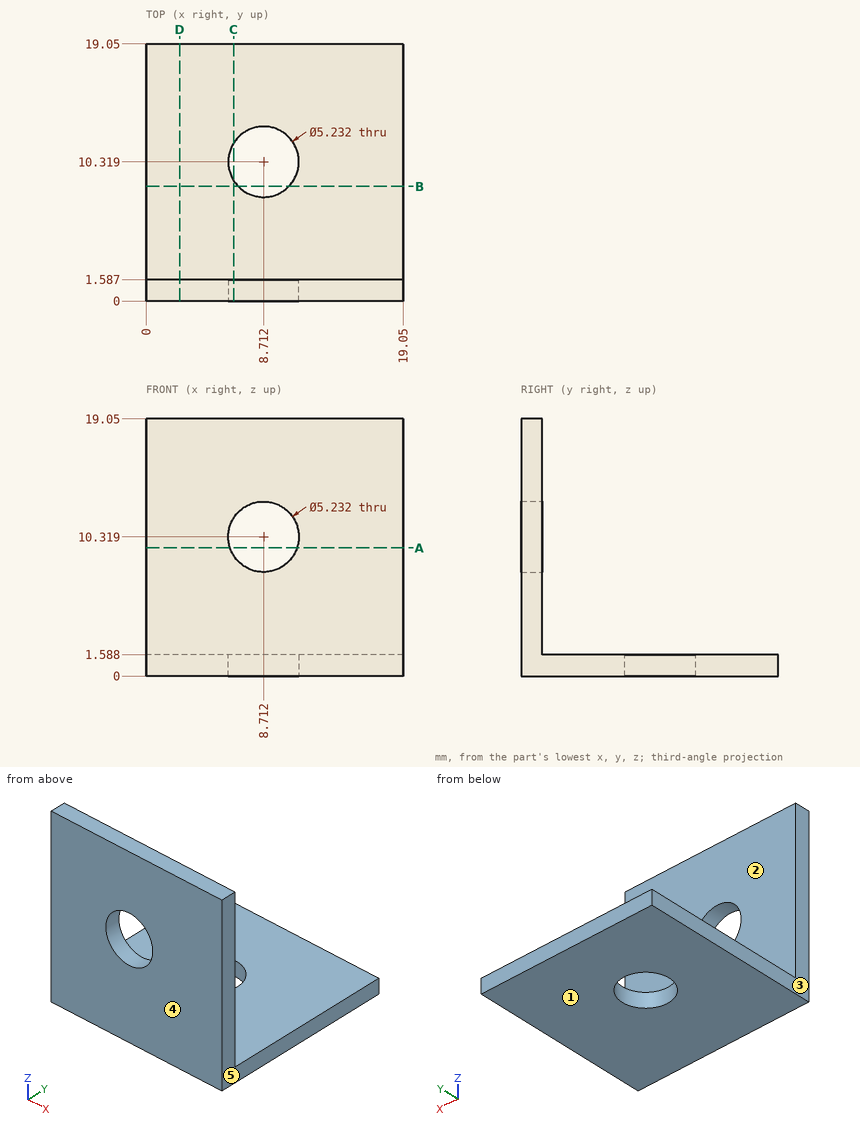
Part print with two shaded views. Sizes in mm from the minimum x, y, z corner. A direction names the side the tool comes from. Round coordinates to 2 decimals unless told otherwise and drop trailing zeros. Order: outer loops, then holes, each group sorted by start corner. A loop starts at its lowest first (then second) coordinate and runs counter-clockwise, first axis right, second up. Notation, with made-up numbers: (43.25, 35.5) -> (89.25, 35.5) arc R23 ccw to (89.25, 57.5) -> close; hole circle Ø7 at (13.25, 21.5). An arc over 180 degrees is marked (long way). One line per question, with ' | ' between items.
Q1. Slice it at A-A (z = 9.5). Write the cut outline in (x, y).
Completed:
outline: (0, 0) -> (6.23, 0) -> (6.23, 1.59) -> (0, 1.59) -> close; (11.2, 0) -> (19.05, 0) -> (19.05, 1.59) -> (11.2, 1.59) -> close
Q2. Slice it at C-C (x = 6.5). Give the number of separate pieces and of enclosed holes in the cut face.
Completed:
separate pieces: 3 | enclosed holes: 0
Q3. Slice it at D-D (x = 2.5). Write the cut outline in (y, z).
Completed:
outline: (0, 0) -> (19.05, 0) -> (19.05, 1.59) -> (1.59, 1.59) -> (1.59, 19.05) -> (0, 19.05) -> close
Q4. Drop flat-ended pins along their axis: pin 1 (8.5 mm diameter, centred on x = 13, y = 11, fed in from +Z); pin 2 (6 mm diameter, centred on x = 15, z = 12.5, fed in from +Y). Give the stop position or say it passes through.
Completed:
pin 1: stops at z = 1.59 | pin 2: stops at y = 1.59
Q5. Two-plate mould, pull along X, no slides. Class the marked faces 3, 4 and 5: released by +X, released by -X, zero draft, split by the parting line, or undercut.
Completed:
face 3: released by -X | face 4: zero draft | face 5: released by +X
Q6. Slice it at B-B (y = 8.5). Write the cut outline in (x, z).
Completed:
outline: (0, 0) -> (6.83, 0) -> (6.83, 1.59) -> (0, 1.59) -> close; (10.59, 0) -> (19.05, 0) -> (19.05, 1.59) -> (10.59, 1.59) -> close
Q7. Which spindle directions (+Z, -Z, +X, -X, +Y, -Y) get a long thin tool onto all of the face, cutting with end or side? Do the marked faces 1 and 2. Say none if no direction does.
Completed:
face 1: -Z, +X, -X, +Y, -Y | face 2: +Z, +X, -X, +Y
Q8. Probe probe 1 along Z at (x, y) = (5.5, 3.75). List the from-to ranges inside material, lowest first.
Completed:
probe 1: z = 0 to 1.59
